```python
from build123d import *

# Parameters (mm, degrees)
SKETCH_2_W          = 65.7
SKETCH_2_H          = 30
EXTRUDE_1_DEPTH     = 4
FILLET_1_R          = 2
SKETCH_5_R          = 1.1
SKETCH_5_W          = 1.5
SKETCH_5_H          = 16
CUT_EXTRUDE_6_DEPTH = 37.333490061
SKETCH_3_W          = 4.8
SKETCH_3_H          = 4.45
SKETCH_3_R          = 1.1
CUT_EXTRUDE_5_DEPTH = 2.4
FILLET_7_R          = 0.51
FILLET_8_R          = 0.6
FILLET_9_R          = 0.5
FILLET_10_R         = 0.8


with BuildPart() as part:
    # 스케치2 → 보스-돌출1 (new body)
    with BuildSketch(Plane.XY):
        Rectangle(SKETCH_2_W, SKETCH_2_H)
    extrude(amount=EXTRUDE_1_DEPTH)

    # 필렛1
    fillet_1_edges = [part.edges().sort_by_distance(p)[0] for p in [
        (32.85, 15, 2),
        (32.85, -15, 2),
        (-32.85, -15, 2),
        (-32.85, 15, 2),
    ]]
    fillet(fillet_1_edges, radius=FILLET_1_R)

    # 스케치5 → 컷-돌출6 (cut, through all)
    with BuildSketch(Plane.XY.offset(4)):
        with Locations((-29.85, 12.35)):
            Circle(SKETCH_5_R)
        with Locations(Location((29.85, 12.35, 0), (0, 0, 180))):
            Circle(SKETCH_5_R)
        with Locations((29.85, -12.35)):
            Circle(SKETCH_5_R)
        with Locations(Location((-29.85, -12.35, 0), (0, 0, 180))):
            Circle(SKETCH_5_R)
        with Locations((-32.1, 0)):
            Rectangle(SKETCH_5_W, SKETCH_5_H)
        with Locations((32.1, 0)):
            Rectangle(SKETCH_5_W, SKETCH_5_H)
    extrude(amount=-CUT_EXTRUDE_6_DEPTH, mode=Mode.SUBTRACT)

    # 스케치3 → 컷-돌출5 (cut)
    # profile 1 of 4: a face of its own
    with BuildSketch(Plane.XY.offset(4)):
        with Locations((-30.45, 12.775)):
            Rectangle(SKETCH_3_W, SKETCH_3_H)
        with Locations((-29.85, 12.35)):
            Circle(SKETCH_3_R, mode=Mode.SUBTRACT)
    # profile 2 of 4: a face of its own
    with BuildSketch(Plane.XY.offset(4)):
        with Locations((-30.45, -12.775)):
            Rectangle(SKETCH_3_W, SKETCH_3_H)
        with Locations(Location((-29.85, -12.35, 0), (0, 0, 180))):
            Circle(SKETCH_3_R, mode=Mode.SUBTRACT)
    # profile 3 of 4: a face of its own
    with BuildSketch(Plane.XY.offset(4)):
        with Locations((30.45, -12.775)):
            Rectangle(SKETCH_3_W, SKETCH_3_H)
        with Locations((29.85, -12.35)):
            Circle(SKETCH_3_R, mode=Mode.SUBTRACT)
    # profile 4 of 4: a face of its own
    with BuildSketch(Plane.XY.offset(4)):
        with Locations((30.45, 12.775)):
            Rectangle(SKETCH_3_W, SKETCH_3_H)
        with Locations(Location((29.85, 12.35, 0), (0, 0, 180))):
            Circle(SKETCH_3_R, mode=Mode.SUBTRACT)
    extrude(amount=-CUT_EXTRUDE_5_DEPTH, mode=Mode.SUBTRACT)

    # 필렛7
    fillet_7_edges = [part.edges().sort_by_distance(p)[0] for p in [
        (-32.85, -10.55, 2.8),
        (-28.05, -15, 2.8),
        (28.05, -15, 2.8),
        (32.85, -10.55, 2.8),
        (32.85, 10.55, 2.8),
        (28.05, 15, 2.8),
        (-28.05, 15, 2.8),
        (-32.85, 10.55, 2.8),
    ]]
    fillet(fillet_7_edges, radius=FILLET_7_R)

    # 필렛8
    fillet_8_edges = [part.edges().sort_by_distance(p)[0] for p in [
        (28.05, -10.55, 2.8),
        (28.05, 10.55, 2.8),
        (-28.05, 10.55, 2.8),
    ]]
    fillet(fillet_8_edges, radius=FILLET_8_R)

    # 필렛9
    fillet_9_edges = [part.edges().sort_by_distance(p)[0] for p in [
        (32.85, 8, 2),
        (32.85, -8, 2),
        (-32.85, -8, 2),
        (-32.85, 8, 2),
    ]]
    fillet(fillet_9_edges, radius=FILLET_9_R)

    # 필렛10
    fillet_10_edges = [part.edges().sort_by_distance(p)[0] for p in [
        (31.35, 8, 2),
        (31.35, -8, 2),
        (-31.35, 8, 2),
        (-31.35, -8, 2),
    ]]
    fillet(fillet_10_edges, radius=FILLET_10_R)


solid = part.part
```
Build history of the part. All positions in model axes, mm. A direction names the side the tool comes from. Round coordinates to 2 decimals unless told otherwise and drop trailing zeros. Loops run counter-clockwise (first coordinate to the right, second up) from the corner with the lowest first, then second, coordinate; pieces in that order, holes last. Notation, with made-up numbers: M -39.5,-12.5 L -27.5,-12.5 A5 cw -27.5,-5.5 Z; hole C 32,2.25 d2. An arc over 180 degrees is marked long. Answer as CSV lines item,"result".
1. 3-axis set-ups, long thin cutter, end or side, ignore diameter. For faces 1 (the flat face through (-31, -13, 1.6)), 2 (the flat face through (0, -15, 2)), 3 (the flat face through (30, -10.55, 3)), 4 (the flat face through (30, 10.55, 3)), 5 (the flat face through (31.35, 0, 2)): which of +Z, -Z, +X, -X, +Y, -Y reach the whole face in a straight line?
Resolved:
face 1,"+Z, -X, -Y"
face 2,"+Z, -Z, +X, -X, -Y"
face 3,"+Z, +X, -Y"
face 4,"+Z, +X, +Y"
face 5,"+Z, -Z, +X"
2. Cut at C-C on z = 0.7. Write the cut outline in (x, y), then the cut area to 3 significant figures.
Resolved:
outline,"M -32.85,-13 A2 ccw -30.85,-15 L 30.85,-15 A2 ccw 32.85,-13 L 32.85,-8.5 A0.5 ccw 32.35,-8 L 32.15,-8 A0.8 cw 31.35,-7.2 L 31.35,7.2 A0.8 cw 32.15,8 L 32.35,8 A0.5 ccw 32.85,8.5 L 32.85,13 A2 ccw 30.85,15 L -30.85,15 A2 ccw -32.85,13 L -32.85,8.5 A0.5 ccw -32.35,8 L -32.15,8 A0.8 cw -31.35,7.2 L -31.35,-7.2 A0.8 cw -32.15,-8 L -32.35,-8 A0.5 ccw -32.85,-8.5 Z; hole C -29.85,-12.35 d2.2; hole C -29.85,12.35 d2.2; hole C 29.85,-12.35 d2.2; hole C 29.85,12.35 d2.2"
area,"1,900 mm²"
3. Flat gauge pins, fed straight in: P1, Ø2.5, axis at x = 29.85, y = -12.35, coming from the +Z side; P2, Ø1.2, axis at y = 0.5, z = 1, coming from the +X side; P3, Ø0.7, axis at x = 31, z = 3, coming from the +Y side. Where does each tip first touch, or does it go through?
Resolved:
P1,"stops at z = 1.6"
P2,"stops at x = 31.35"
P3,"stops at y = 10.55"
4. Cut at D-D on y = 3.25. Write the cut outline in (x, z).
Resolved:
outline,"M -31.35,0 L 31.35,0 L 31.35,4 L -31.35,4 Z"
5. Cut at B-B on y = 12.35. Write the cut outline in (x, z).
Resolved:
outline,"M -32.85,0 L -30.95,0 L -30.95,1.6 L -32.85,1.6 Z; M -28.75,0 L 28.75,0 L 28.75,1.6 L 28.05,1.6 L 28.05,4 L -28.05,4 L -28.05,1.6 L -28.75,1.6 Z; M 30.95,0 L 32.85,0 L 32.85,1.6 L 30.95,1.6 Z"
6. Wall check: probe 1 along Y at (x, z) = (29.85, 1.25); probe 2 along X at (y, z) = (6.5, 1.6); probe 3 along X at (y, z) = (12, 1.35). Give the ranges that are in metal, low to high. Write a range as [from, to].
Resolved:
probe 1,"y = [-15, -13.45], [-11.25, 11.25], [13.45, 15]"
probe 2,"x = [-31.35, 31.35]"
probe 3,"x = [-32.85, -30.89], [-28.81, 28.81], [30.89, 32.85]"
7. Two-plate mould, pull along X, no slides. Class faces 6 (the flat face through (-28.05, 13, 3)), 7 (the flat face through (0, 15, 2)), 8 (the cylindrical face through (-30.95, 12.4, 0.81)): released by +X, released by -X, zero draft, split by the parting line, or undercut.
Resolved:
face 6,"released by -X"
face 7,"zero draft"
face 8,"undercut"
8. Cut at A-A on x = -29.85. Write the cut outline in (y, z), then the cut area to 3 significant figures.
Resolved:
outline,"M -15,0 L -13.45,0 L -13.45,1.6 L -15,1.6 Z; M -11.25,0 L 11.25,0 L 11.25,1.6 L 10.55,1.6 L 10.55,4 L -10.55,4 L -10.55,1.6 L -11.25,1.6 Z; M 13.45,0 L 15,0 L 15,1.6 L 13.45,1.6 Z"
area,"91.6 mm²"
